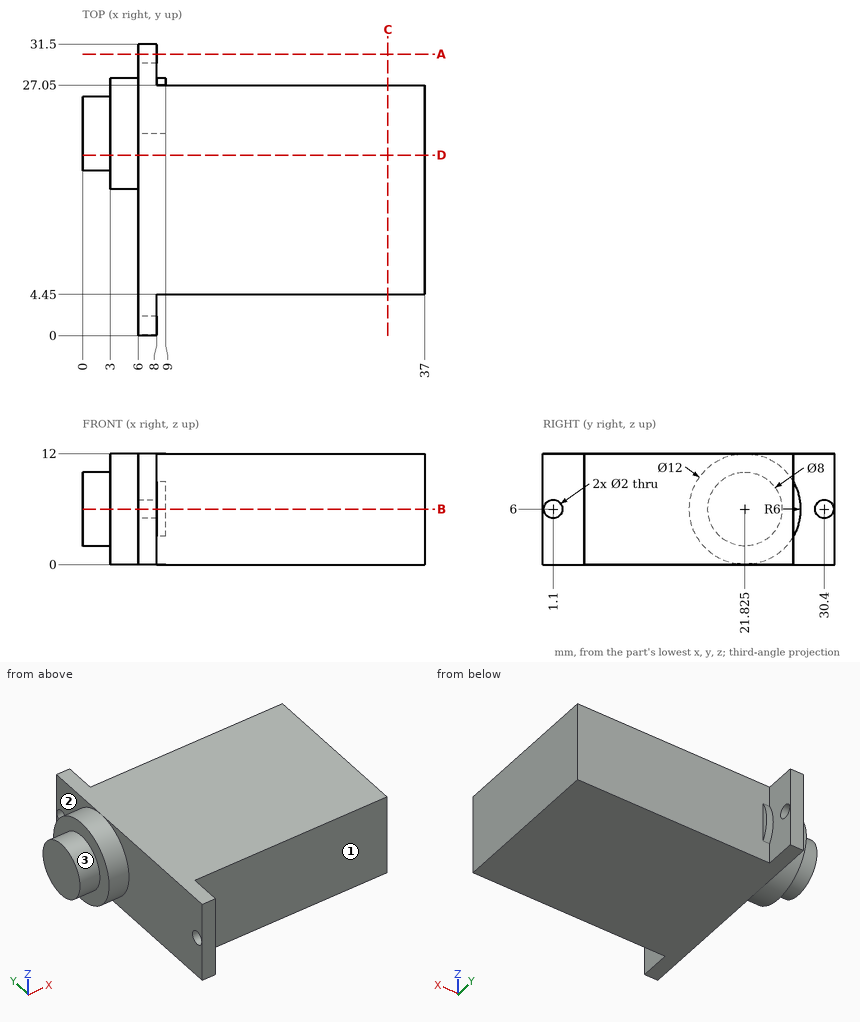
Here's the drawing with two shaded views (mm, measured from the low corner). I have some questions. A direction names the side the tool comes from. Give positions to 0.01 mm unless a question says otherwise; leave off trailing zeros. Order: outer loops, then holes, each group sorted by start corner. A loop starts at its lowest first (then second) coordinate and runs counter-clockwise, first axis right, second up. Notation, with made-up numbers: M 9,-19 L 61,-19 A14 ccw 61,2 Z; hole C 54.25,48.5 d3. An arc over 180 degrees is marked long. One line per item, written item: value.
1) For P1, Ø1.5, axis at y = 13, z = 6.5, coming from the -X side; P2, Ø5, axis at y = 1, z = 6.5, coming from the +X side; P3, Ø2, axis at x = 13, z = 10, coming from the -Y side; P4, Ø1.6, axis at y = 30.4, z = 6, coming from the -X side, each with a flat end and sliding along its axis, tell me the tip position at first contact or that it passes through.
Answer sheet:
P1: stops at x = 6
P2: stops at x = 8
P3: stops at y = 4.45
P4: passes through
2) I want a section at D-D, the plane y = 19.5. List the corners of the cut face in (x, z) for me (1 decimal), plus the area to 3 significant figures.
Answer sheet:
outline: M 0,2.7 L 3,2.7 L 3,0.5 L 6,0.5 L 6,0 L 37,0 L 37,12 L 6,12 L 6,11.5 L 3,11.5 L 3,9.3 L 0,9.3 Z
area: 425 mm^2
3) I want a section at B-B, the plane z = 6. Count the separate pieces of the cut face and the enclosed holes in it, plus the area to 3 significant figures.
Answer sheet:
separate pieces: 3
enclosed holes: 0
area: 771 mm^2
4) Please list where these lines run through material, in increasing order: line 1 along X through (y, z) = (10, 4.25); line 2 along Y through (x, z) = (29, 8.5); line 3 along X through (y, z) = (3.5, 2).
Answer sheet:
line 1: x = 6 to 37
line 2: y = 4.45 to 27.05
line 3: x = 6 to 8
5) On a 3-axis mill with a long thin cutter (end or side, diameter ignored), from which of +Z, -Z, +X, -X, +Y, -Y can I reach the whole of each face in a straight line? I mean the marked faces 1, 2 and 3. Say none if no direction works.
Answer sheet:
face 1: +Z, -Z, +X, -Y
face 2: -X, +Y
face 3: -X
6) I want a section at C-C, the plane x = 33. List the corners of the cut face in (y, z) for me, plus the area to 3 significant figures.
Answer sheet:
outline: M 4.45,0 L 27.05,0 L 27.05,12 L 4.45,12 Z
area: 271 mm^2
7) I want a section at A-A, the plane y = 30.4. List the corners of the cut face in (x, z) for me.
Answer sheet:
outline: M 6,0 L 8,0 L 8,5 L 6,5 Z; M 6,7 L 8,7 L 8,12 L 6,12 Z
